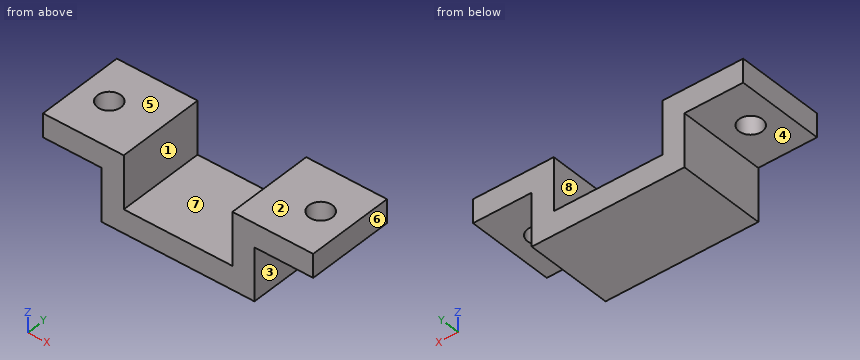
from build123d import *

# Parameters (mm, degrees)
F0_W     = 46
F0_H     = 15
F1_DEPTH = 13
F2_W     = 18.5
F2_H     = 15
F3_DEPTH = 9
F4_W     = 10
F4_H     = 15
F5_DEPTH = 9
F6_R     = 2
F7_DEPTH = 25


with BuildPart() as f1:
    # F0 (on Top) → F1 (new body)
    with BuildSketch(Plane.XY):
        Rectangle(F0_W, F0_H)
    extrude(amount=F1_DEPTH)

    # F2 (on face) → F3 (cut)
    with BuildSketch(Plane.XY.offset(13)):
        Rectangle(F2_W, F2_H)
    extrude(amount=-F3_DEPTH, mode=Mode.SUBTRACT)

    # F4 (on face) → F5 (cut)
    with BuildSketch(Plane(origin=(0, 0, 0), x_dir=(1, 0, 0), z_dir=(0, 0, -1))):
        with Locations((-18, 0)):
            Rectangle(F4_W, F4_H)
        with Locations((18, 0)):
            Rectangle(F4_W, F4_H)
    extrude(amount=-F5_DEPTH, mode=Mode.SUBTRACT)

    # F6 (on face) → F7 (cut)
    with BuildSketch(Plane(origin=(0, 0, 9), x_dir=(1, 0, 0), z_dir=(0, 0, -1))):
        with Locations((-18, 0)):
            Circle(F6_R)
        with Locations((18, 0)):
            Circle(F6_R)
    extrude(amount=-F7_DEPTH, mode=Mode.SUBTRACT)


solid = f1.part
The listing builds one solid part. Answer for the finished solid, in the listing's coordinates (mm). Face numbers are marked on the shaded views. A direction names the side the tool comes from. Round coordinates to 2 decimals unless told otherwise and drop trailing zeros. Loops run counter-clockwise (first coordinate to the right, second up) from the corner with the lowest first, then second, coordinate; pieces in that order, holes last. Notation, with made-up numbers: M 41.25,-11.5 L 54.25,-11.5 A15 ccw 54.25,-4.5 Z; hole C 64,-22 d1. An arc over 180 degrees is marked long. Return JSON: item names as keys, results as strings.
Q1. Each of these flat-tipped pins is pushed along its axis until it touches: pin 1 Ø4.5 at (y, z) = (3.5, 6) entering from -X; pin 2 Ø4.5 at (x, y) = (2, -0.5) entering from +Z; pin 3 Ø5 at (x, y) = (18.5, -3) entering from -Z; pin 4 Ø3 at (x, y) = (18, 0) entering from -Z. Where does it stop, or does it pass through?
Results list:
{"pin 1": "stops at x = -13", "pin 2": "stops at z = 4", "pin 3": "stops at z = 9", "pin 4": "passes through"}
Q2. Find section A-A, the plane z = 7. Determine the outline of the cut face in (x, y).
Results list:
{"outline": "M -13,-7.5 L -9.25,-7.5 L -9.25,7.5 L -13,7.5 Z; M 9.25,-7.5 L 13,-7.5 L 13,7.5 L 9.25,7.5 Z"}
Q3. Which of the six approach directions +Z, -Z, +X, -X, +Y, -Y give full straight-line access (tool end or side, diameter ignored) to the marked faces 1, 2, 3 and 4?
Results list:
{"face 1": "+Z, +Y, -Y", "face 2": "+Z, +X, -X, +Y, -Y", "face 3": "-Z, +X, +Y, -Y", "face 4": "-Z, -X, +Y, -Y"}
Q4. The mould has two halves that part along X. Classify the marked faces 5, 6, 7 and 8: released by +X, released by -X, zero draft, split by the parting line, or undercut.
Results list:
{"face 5": "zero draft", "face 6": "released by +X", "face 7": "undercut", "face 8": "undercut"}
Q5. Find section B-B, the plane x = -18. Determine the outline of the cut face in (y, z).
Results list:
{"outline": "M -7.5,9 L -2,9 L -2,13 L -7.5,13 Z; M 2,9 L 7.5,9 L 7.5,13 L 2,13 Z"}
Q6. Find section C-C, the plane y = 0. Determine the outline of the cut face in (x, z), plus the area to 4 significant figures.
Results list:
{"outline": "M -23,9 L -20,9 L -20,13 L -23,13 Z; M -16,9 L -13,9 L -13,0 L 13,0 L 13,9 L 16,9 L 16,13 L 9.25,13 L 9.25,4 L -9.25,4 L -9.25,13 L -16,13 Z; M 20,9 L 23,9 L 23,13 L 20,13 Z", "area": "219.5 mm2"}
Q7. Find the intervals of material crossed by line 1 along X through (y, z) = (0, 11.2); line 2 along X through (y, z) = (3.75, 6); line 3 along Y through (x, z) = (18, 10.35), in increasing order. Write a range as from..to.
Results list:
{"line 1": "x = -23..-20, -16..-9.25, 9.25..16, 20..23", "line 2": "x = -13..-9.25, 9.25..13", "line 3": "y = -7.5..-2, 2..7.5"}
Q8. Find section D-D, the plane y = -4.75. Determine the outline of the cut face in (x, z).
Results list:
{"outline": "M -23,9 L -13,9 L -13,0 L 13,0 L 13,9 L 23,9 L 23,13 L 9.25,13 L 9.25,4 L -9.25,4 L -9.25,13 L -23,13 Z"}
